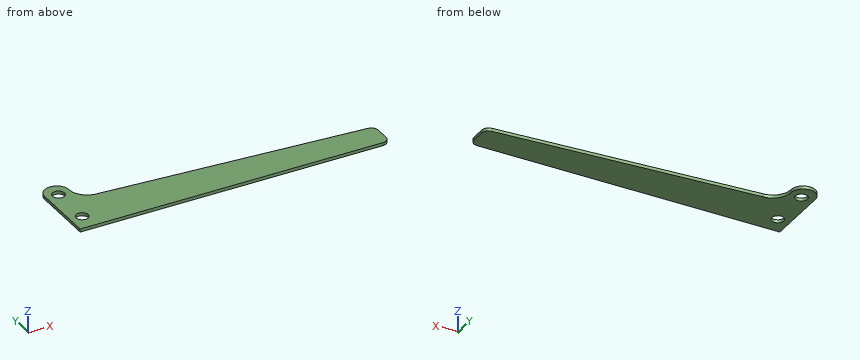
from build123d import *

# Parameters (mm, degrees)
SKETCH1_R           = 1.5875
BOSS_EXTRUDE1_DEPTH = 0.8128


with BuildPart() as part:
    # Sketch1 → Boss-Extrude1 (new body)
    with BuildSketch(Plane.XY):
        with BuildLine():
            Line((0, -0.8128), (79.461894979, -0.8128))
            ThreePointArc((79.461894979, -0.8128), (80.749213577, -0.279575177), (81.2824384, 1.007743421))
            Line((81.2824384, 1.007743421), (81.2824384, 4.648830263))
            ThreePointArc((81.2824384, 4.648830263), (80.792085251, 5.891799366), (79.585173538, 6.465194969))
            Line((79.585173538, 6.465194969), (11.1125, 11.1125))
            ThreePointArc((11.1125, 11.1125), (7.744903955, 12.507403955), (6.35, 15.875))
            ThreePointArc((6.35, 15.875), (3.175, 19.05), (0, 15.875))
            Line((0, 15.875), (0, -0.8128))
        make_face()
        with Locations((3.175, 3.96875)):
            Circle(SKETCH1_R, mode=Mode.SUBTRACT)
        with Locations((3.175, 15.08125)):
            Circle(SKETCH1_R, mode=Mode.SUBTRACT)
    extrude(amount=BOSS_EXTRUDE1_DEPTH)


solid = part.part
For this review, take the finished solid that the model builds, in its own axes (mm). Round coordinates to 2 decimals unless told otherwise and drop trailing zeros. Order: outer loops, then holes, each group sorted by start corner. A loop starts at its lowest first (then second) coordinate and runs counter-clockwise, first axis right, second up. Notation, with made-up numbers: M 80,-14 L 89,-14 A30 cw 89,12 Z; hole C 84.5,89.5 d10. An arc over 180 degrees is marked long. Use a Markdown table: item, result. Add a question column.
Item 1: Add section B-B, the plane y = 3.25. Give the boundary of the cut face in (x, z), then the cut area to 3 significant figures.
Item 2: To check wall thickness, follow line 1 along X through (y, z) = (15.75, 0.35); line 2 along X through (y, z) = (4.25, 0.5); line 3 along Y through (x, z) = (37.5, 0.65). State the ranges of each line that lie inside material, in increasing order.
Item 3: Add section C-C, the plane x = 48. Give the boundary of the cut face in (y, z), then the cut area to 3 significant figures.
Item 4: Add section A-A, the plane z = 0.2. State how many separate pieces and enclosed holes the cut face has, then the cut area to 3 significant figures.
Item 5: Add section D-D, the plane y = 17.5. Give the boundary of the cut face in (x, z).
Geometry results:
| question | item | result |
|---|---|---|
| 1 | outline | M 0,0 L 1.76,0 L 1.76,0.81 L 0,0.81 Z; M 4.59,0 L 81.28,0 L 81.28,0.81 L 4.59,0.81 Z |
| 1 | area | 63.8 mm² |
| 2 | line 1 | x = 0 to 1.74, 4.61 to 6.35 |
| 2 | line 2 | x = 0 to 1.61, 4.74 to 81.28 |
| 2 | line 3 | y = -0.81 to 9.32 |
| 3 | outline | M -0.81,0 L 8.61,0 L 8.61,0.81 L -0.81,0.81 Z |
| 3 | area | 7.66 mm² |
| 4 | separate pieces | 1 |
| 4 | enclosed holes | 2 |
| 4 | area | 836 mm² |
| 5 | outline | M 0.45,0 L 5.9,0 L 5.9,0.81 L 0.45,0.81 Z |
